```python
from build123d import *

# Parameters (mm, degrees)
SKETCH2_R           = 10
BOSS_EXTRUDE1_DEPTH = 80
SKETCH4_W           = 20
SKETCH4_H           = 40
CUT_EXTRUDE1_DEPTH  = 139.564064606
FILLET1_R           = 3
FILLET2_R           = 3
CHAMFER1_SIZE       = 10
CHAMFER2_SIZE       = 10
CHAMFER3_SIZE       = 10
FILLET4_R           = 3
FILLET5_R           = 3
FILLET6_R           = 3


with BuildPart() as part:
    # Sketch2 → Boss-Extrude1 (new body)
    with BuildSketch(Plane(origin=(0, 0, 0), x_dir=(1, 0, 0), z_dir=(0, 1, 0))):
        Polygon((0, 0), (-80, 0), (-80, 40), (-40, 40), (-40, 80), (0, 80), align=None)
        with Locations(Location((-20, 20, 0), (0, 0, 270))):
            Circle(SKETCH2_R, mode=Mode.SUBTRACT)
    extrude(amount=BOSS_EXTRUDE1_DEPTH)

    # Sketch4 → Cut-Extrude1 (cut, through all)
    with BuildSketch(Plane(origin=(0, 0, 0), x_dir=(0, 0, -1), z_dir=(1, 0, 0))):
        with Locations((70, 40)):
            Rectangle(SKETCH4_W, SKETCH4_H)
    extrude(amount=-CUT_EXTRUDE1_DEPTH, mode=Mode.SUBTRACT)

    # Fillet1
    fillet1_edges = [part.edges().sort_by_distance(p)[0] for p in [
        (-20, 0, -80),
    ]]
    fillet(fillet1_edges, radius=FILLET1_R)

    # Fillet2
    fillet2_edges = [part.edges().sort_by_distance(p)[0] for p in [
        (-20, 80, -80),
    ]]
    fillet(fillet2_edges, radius=FILLET2_R)

    # Chamfer1
    chamfer1_edges = [part.edges().sort_by_distance(p)[0] for p in [
        (-20, 60, -80),
    ]]
    chamfer(chamfer1_edges, length=CHAMFER1_SIZE)

    # Chamfer2
    chamfer2_edges = [part.edges().sort_by_distance(p)[0] for p in [
        (-20, 20, -80),
    ]]
    chamfer(chamfer2_edges, length=CHAMFER2_SIZE)

    # Chamfer3
    chamfer3_edges = [part.edges().sort_by_distance(p)[0] for p in [
        (-80, 40, -40),
    ]]
    chamfer(chamfer3_edges, length=CHAMFER3_SIZE)

    # Fillet4
    fillet4_edges = [part.edges().sort_by_distance(p)[0] for p in [
        (-40, 40, -40),
    ]]
    fillet(fillet4_edges, radius=FILLET4_R)

    # Fillet5
    fillet5_edges = [part.edges().sort_by_distance(p)[0] for p in [
        (-20, 0, -30),
    ]]
    fillet(fillet5_edges, radius=FILLET5_R)

    # Fillet6
    fillet6_edges = [part.edges().sort_by_distance(p)[0] for p in [
        (-20, 80, -30),
    ]]
    fillet(fillet6_edges, radius=FILLET6_R)


solid = part.part
```
Verification items for the finished model (mm, model axes). A direction names the side the tool comes from. Round coordinates to 2 decimals unless told otherwise and drop trailing zeros. Write each loop counter-clockwise with the first axis right and the second up, starting at its lowest first coordinate (ties: lowest second). Pieces come first, ordered by that corner, then holes.
1. Scan lines: L1, parallel to X at y = 19, z = -20; L2, parallel to Z at x = -49.5, y = 22; L3, parallel to Z at x = -31.5, y = 34. Record each from-to range of solid material in increasing order.
2. Draft check along Y on faces 4 (the flat face through (-57, 39, -40)), 5 (the flat face through (-20, 65, -75)), 6 (the cylindrical face through (-19.72, 79.14, -79.1)). Enter one of: +Y half, -Y half, draft (parallel to the pull), parting line (faces both ways), or undercut.
3. Section check A-A on z = -65. Enter the section's corners in (x, y).
4. Section check C-C on x = -20. Enter the section's corners in (y, z).
5. Section check D-D on z = -20. Enter the section's corners in (x, y).
6. Access from +Z, -Z, +X, -X, +Y, -Y to the whole of each face (thin tool, end or side, straight path). Record for faces 1 (the flat face through (-20, 40, -60)), 2 (the flat face through (-39, 39, 0)), 3 (the flat face through (-40, 39, -57)).
7. Gauge pin test, flat ends, axial feed: P1, Ø8, axis at x = -51.5, y = 59.5, coming from the -Z side; P2, Ø5, axis at x = -19.5, y = 28, coming from the -Z side; P3, Ø1, axis at x = -21, y = 69, coming from the -Z side; P4, Ø1.5, axis at y = 72, z = -50, coming from the +X side. Record the tip position at first contact, or that the pin passes through.
8. Section check B-B on y = 6. Enter the section's corners in (x, z).
Answer:
1. L1: x = -80 to -30, -10 to 0
1. L2: z = -40 to 0
1. L3: z = -60 to 0
2. face 4: draft
2. face 5: undercut
2. face 6: +Y half
3. outline: (-40, 0) - (0, 0) - (0, 20) - (-40, 20) - close; (-40, 60) - (0, 60) - (0, 80) - (-40, 80) - close
4. outline: (0, -77) arc R3 ccw to (3, -80) - (10, -80) - (20, -70) - (20, -60) - (60, -60) - (60, -70) - (70, -80) - (77, -80) arc R3 ccw to (80, -77) - (80, -33) arc R3 ccw to (77, -30) - (3, -30) arc R3 ccw to (0, -33) - close; (0, -7) arc R3 ccw to (3, -10) - (77, -10) arc R3 ccw to (80, -7) - (80, 0) - (0, 0) - close
5. outline: (-80, 0) - (-33, 0) arc R3 ccw to (-30, 3) - (-30, 77) arc R3 ccw to (-33, 80) - (-80, 80) - close; (-10, 3) arc R3 ccw to (-7, 0) - (0, 0) - (0, 80) - (-7, 80) arc R3 ccw to (-10, 77) - close
6. face 1: -Z, +X, -X
6. face 2: +Z, +X, -X, +Y, -Y
6. face 3: -Z, -X, +Y, -Y
7. P1: stops at z = -40
7. P2: stops at z = -60
7. P3: stops at z = -79.5
7. P4: stops at x = 0
8. outline: (-80, -30) - (-70, -40) - (-43, -40) arc R3 cw to (-40, -43) - (-40, -80) - (0, -80) - (0, 0) - (-80, 0) - close; hole circle Ø20 at (-20, -20)
